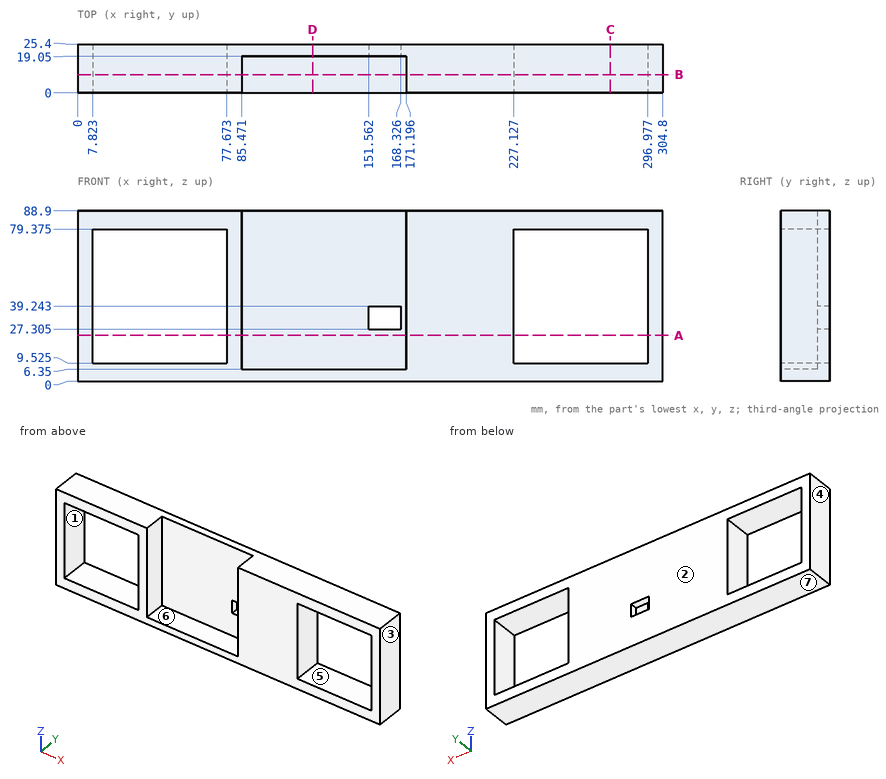
The drawing under review shows one solid part. Ordinate dimensions are in mm from its lowest x, y, z. A direction names the side the tool comes from. Round coordinates to 2 decimals unless told otherwise and drop trailing zeros. Order: outer loops, then holes, each group sorted by start corner. A loop starts at its lowest first (then second) coordinate and runs counter-clockwise, first axis right, second up. Notation, with made-up numbers: M -19,41.5 L -10,41.5 A21 cw -10,80.5 Z; hole C -36.75,-13.5 d11. An arc over 180 degrees is marked long. Answer as CSV lines item,"result". Start each with the question number.
1) Wall thickness on line 1 along X through (y, z) = (20.75, 59); line 2 along X through (y, z) = (3, 26.5); line 3 along Z through (x, y) = (283, 9.75) (3 decimals): over which ranges is each line inside the solid? List them lowest first. Write a range as [from, to].
2) The part is to be moulded in two halves that separate along X. For the marked faces 1, 2, 3 and 4, say which applies: +X half, -X half, draft (parallel to the pull), parting line (faces both ways), or undercut.
3) Add section D-D (x = 122.5). Give the boundary of the cut face in (y, z).
4) Add section B-B (y = 9.5). Give the number of separate pieces and of enclosed holes in the cut face, then the cut area to 3 significant figures.
5) Add section C-C (x = 277.5). Give the boundary of the cut face in (y, z) (3 decimals).
6) Tool access review of the marked faces 5, 6 and 7: name each direction out of +Z, -Z, +X, -X, +Y, -Y from which nothing blocks a thin tool from reaching the whole face with its end or side.
7) Add section A-A (z = 24). Give the boundary of the cut face in (x, y).
8) For pin 1 Ø3 at (x, y) = (134.5, 5.5) entering from -Z; pin 2 Ø25 at (x, z) = (127.5, 42.5) entering from -Y, all flat-tipped, find the tip position at first contact; note any pin that passes through.
Resolved:
1,line 1,"[0, 7.82], [77.67, 227.13], [296.98, 304.8]"
1,line 2,"[0, 7.82], [77.67, 85.47], [171.2, 227.13], [296.98, 304.8]"
1,line 3,"[0, 9.525], [79.375, 88.9]"
2,face 1,"undercut"
2,face 2,"draft"
2,face 3,"+X half"
2,face 4,"-X half"
3,outline,"M 0,0 L 25.4,0 L 25.4,88.9 L 19.05,88.9 L 19.05,6.35 L 0,6.35 Z"
4,separate pieces,"1"
4,enclosed holes,"2"
4,area,"10,300 mm^2"
5,outline,"M 0,0 L 25.4,0 L 25.4,9.525 L 0,9.525 Z; M 0,79.375 L 25.4,79.375 L 25.4,88.9 L 0,88.9 Z"
6,face 5,"+Y, -Y"
6,face 6,"+Z, -Y"
6,face 7,"-Z, +X, -X, +Y, -Y"
7,outline,"M 0,0 L 7.82,0 L 7.82,25.4 L 0,25.4 Z; M 77.67,0 L 85.47,0 L 85.47,19.05 L 171.2,19.05 L 171.2,0 L 227.13,0 L 227.13,25.4 L 77.67,25.4 Z; M 296.98,0 L 304.8,0 L 304.8,25.4 L 296.98,25.4 Z"
8,pin 1,"z = 0"
8,pin 2,"y = 19.05"
